```python
from build123d import *

# Parameters (mm, degrees)
SKETCH1_R                                            = 1.0000000000000033
SKETCH1_R_2                                          = 0.9999999999999979
SKETCH1_R_3                                          = 1.000000000000005
SKETCH1_R_4                                          = 1.0000000000000018
SKETCH1_R_5                                          = 1.0000000000000029
MAIN_BODY_DEPTH                                      = 10.5
PROFILE_STOPS_DEPTH                                  = 20
CSK_FOR_M3_HEX_SOCKET_COUNTERSUNK_HEAD_S_D           = 3.2
CSK_FOR_M3_HEX_SOCKET_COUNTERSUNK_HEAD_S_DEPTH       = 30.5
CSK_FOR_M3_HEX_SOCKET_COUNTERSUNK_HEAD_S_CSINK_D     = 6.94
CSK_FOR_M3_HEX_SOCKET_COUNTERSUNK_HEAD_S_CSINK_ANGLE = 90
CSK_FOR_M5_HEX_SOCKET_COUNTERSUNK_HEAD_S_D           = 5.3
CSK_FOR_M5_HEX_SOCKET_COUNTERSUNK_HEAD_S_DEPTH       = 30.5
CSK_FOR_M5_HEX_SOCKET_COUNTERSUNK_HEAD_S_CSINK_D     = 11.47
CSK_FOR_M5_HEX_SOCKET_COUNTERSUNK_HEAD_S_CSINK_ANGLE = 90
FILLET1_R                                            = 5
FILLET3_R                                            = 5
DRAFT1_ANGLE                                         = 0.5000000000000011
CHAMFER2_SIZE                                        = 0.5


with BuildPart() as part:
    # Sketch1 → Main Body (new body)
    with BuildSketch(Plane(origin=(0, 0, 0), x_dir=(1, 0, 0), z_dir=(0, 1, 0))):
        Polygon((-55, 0), (55, -6.74e-15), (-17.37778423417673, 103.36618828645003), align=None)
        with Locations(Location((-1.2076863300743388, 10.249999999999998, 0), (0, 0, 90))):
            Circle(SKETCH1_R, mode=Mode.SUBTRACT)
        with Locations(Location((23.307593201638067, 10.25, 0), (0, 0, 90))):
            Circle(SKETCH1_R_2, mode=Mode.SUBTRACT)
        with Locations(Location((-26.970095805737262, 47.04253374154206, 0), (0, 0, 90))):
            Circle(SKETCH1_R_3, mode=Mode.SUBTRACT)
        with Locations(Location((-18.585376386632234, 70.07936101399606, 0), (0, 0, 90))):
            Circle(SKETCH1_R_4, mode=Mode.SUBTRACT)
        with Locations(Location((2.578216537695586, 40.31670125636554, 0), (0, 0, 90))):
            Circle(SKETCH1_R_5, mode=Mode.SUBTRACT)
    extrude(amount=MAIN_BODY_DEPTH)

    # Sketch1<3> → Profile Stops (add)
    with BuildSketch(Plane(origin=(0, 0, 0), x_dir=(1, 0, 0), z_dir=(0, 1, 0))):
        Polygon((-55, 0), (-24.222965861786736, 0), (-24.22296586178674, 20.499999999999996), (40.64574546670092, 20.500000000000004), (-3.023529700877628, 82.86618828645001), (-25.209935646798243, 21.909538931178865), (-44.47363437290938, 28.920951869355026), align=None)
        Polygon((-7.671783462304414, 33.139573989716), (-10.559339294448062, 34.19055836239805), (-7.671783462304414, 42.1240528086273), (-7.6717834623044165, 50.56670125636553), (-4.598910728953966, 50.56670125636553), (-3.547926356271911, 53.45425708850919), (4.385568089957344, 50.56670125636554), (12.828216537695583, 50.56670125636554), (12.828216537695583, 47.49382852301509), (15.715772369839232, 46.44284415033304), (12.828216537695585, 38.5093497041038), (12.828216537695587, 30.066701256365544), (9.755343804345129, 30.066701256365544), (8.70435943166308, 27.1791454242219), (0.7708649854338496, 30.06670125636554), (-7.671783462304413, 30.06670125636554), align=None, mode=Mode.SUBTRACT)
    extrude(amount=-PROFILE_STOPS_DEPTH)

    # CSK for M3 Hex Socket Countersunk Head Screw1
    with Locations(Plane(origin=(-18.585376387, 10.5, -70.079361014), x_dir=(0, 0, 1), z_dir=(0, 1, 0))):
        with Locations((0, 0), (23.036827272, -8.384719419), (59.829361014, 41.892969589), (59.829361014, 17.377690057)):
            CounterSinkHole(CSK_FOR_M3_HEX_SOCKET_COUNTERSUNK_HEAD_S_D / 2, CSK_FOR_M3_HEX_SOCKET_COUNTERSUNK_HEAD_S_CSINK_D / 2, depth=CSK_FOR_M3_HEX_SOCKET_COUNTERSUNK_HEAD_S_DEPTH, counter_sink_angle=CSK_FOR_M3_HEX_SOCKET_COUNTERSUNK_HEAD_S_CSINK_ANGLE)

    # CSK for M5 Hex Socket Countersunk Head Screw1
    with Locations(Plane(origin=(2.578216538, 10.5, -40.316701256), x_dir=(0, 0, 1), z_dir=(0, 1, 0))):
        with Locations((0, 0)):
            CounterSinkHole(CSK_FOR_M5_HEX_SOCKET_COUNTERSUNK_HEAD_S_D / 2, CSK_FOR_M5_HEX_SOCKET_COUNTERSUNK_HEAD_S_CSINK_D / 2, depth=CSK_FOR_M5_HEX_SOCKET_COUNTERSUNK_HEAD_S_DEPTH, counter_sink_angle=CSK_FOR_M5_HEX_SOCKET_COUNTERSUNK_HEAD_S_CSINK_ANGLE)

    # Fillet1
    fillet1_edges = [part.edges().sort_by_distance(p)[0] for p in [
        (-55, -4.75, 0),
        (-24.222965861786736, -10, 0),
        (-44.47363437290938, -10, -28.920951869355026),
    ]]
    fillet(fillet1_edges, radius=FILLET1_R)

    # Fillet3
    fillet3_edges = [part.edges().sort_by_distance(p)[0] for p in [
        (55, 5.25, 6.74e-15),
        (-17.37778423417673, 5.25, -103.36618828645003),
        (-3.0235297008776296, -10, -82.86618828645001),
        (40.645745466700916, -10, -20.5),
    ]]
    fillet(fillet3_edges, radius=FILLET3_R)

    # Draft1
    draft1_faces = [part.faces().sort_by_distance(p)[0] for p in [
        (11.291780171020358, -10, -30.066701256365544),
        (9.229851618004107, -10, -28.62292334029372),
        (4.737612208548465, -10, -28.622923340293717),
        (-3.4504592384352817, -10, -30.06670125636554),
        (-7.671783462304413, -10.000000000000002, -31.60313762304077),
        (-9.115561378376238, -10, -33.665066176057024),
        (-9.115561378376238, -10, -38.157305585512674),
        (-6.135347095629191, -10, -50.56670125636553),
        (-7.671783462304415, -10, -46.345377032496415),
        (-4.073418542612939, -10, -52.010479172437364),
        (0.4188208668427172, -10, -52.010479172437364),
        (8.606892313826464, -10, -50.56670125636554),
        (12.828216537695583, -10, -49.030264889690315),
        (14.271994453767409, -10, -46.968336336674064),
        (14.271994453767409, -10, -42.476096927218414),
        (12.828216537695587, -10, -34.28802548023467),
    ]]
    draft(draft1_faces, Plane(origin=(0, 0, 0), x_dir=(0, 0, -1), z_dir=(0, -1, 0)), DRAFT1_ANGLE)

    # Chamfer2
    chamfer2_edges = [part.edges().sort_by_distance(p)[0] for p in [
        (-1.232085300572649, 10.5, 3.29e-15),
        (-36.61029010817967, 10.5, -50.52531267809811),
        (-51.95502018773441, 10.5, -2.1321178182447573),
        (18.811107882911628, 10.5, -51.683094143225006),
        (-16.61702500331109, 10.5, -97.58764822980864),
        (49.83014353103527, 10.5, -2.6912569338248247),
    ]]
    chamfer(chamfer2_edges, length=CHAMFER2_SIZE)


solid = part.part
```
The listing builds one solid part. Answer for the finished solid, in the listing's coordinates (mm). A direction names the side the tool comes from. Coordinates: 2 decimals unless noted, no trailing zeros. Write each loop counter-clockwise with the first axis right and the second up, starting at its lowest first coordinate (ties: lowest second). Pieces come first, ordered by that corner, then holes.
Q1. Section D-D, the plane y = 3 is taken. Write down the section's boundary in (x, z), then the cut area to 3 significant figures.
Returned:
outline: (-52.56, -6.71) - (-20.66, -94.34) arc R5 ccw to (-11.87, -95.5) - (49.49, -7.87) arc R5 ccw to (45.4, 0) - (-47.86, 0) arc R5 ccw to start; hole circle Ø3.2 at (-26.97, -47.04); hole circle Ø3.2 at (-18.59, -70.08); hole circle Ø3.2 at (-1.21, -10.25); hole circle Ø5.3 at (2.58, -40.32); hole circle Ø3.2 at (23.31, -10.25)
area: 5,580 mm2
Q2. Which of the six approach directions +Z, -Z, +X, -X, +Y, -Y give full straight-line access (tool end or side, diameter ignored) to faces 1 (the cylindrical face through (35.51, -10.14, -23.26)), 2 (the cylindrical face through (23.38, 4.25, -8.65)), 3 (the flat face through (10, 0, -11)), 4 (the cylindrical face through (-43.65, -10.14, -27.02)), 5 (the flat face through (-9, -20, -30))?
Returned:
face 1: +X, -Y
face 2: +Y, -Y
face 3: +Z, +X, -Y
face 4: -Z, -Y
face 5: +Z, -Z, +X, -X, -Y
Q3. Section C-C, the plane x = 33.5 is taken. Write down the section's boundary in (y, z), then the cut area to 3 significant figures.
Returned:
outline: (-20, -30.71) - (10, -30.71) - (10.5, -29.83) - (10.5, -0.5) - (10, 0) - (0, 0) - (0, -21.15) - (-20, -21.15) - close
area: 513 mm2
Q4. Section B-B, the plane z = -10.25 is taken. Write down the section's boundary in (x, y).
Returned:
outline: (-51.27, -20) - (-24.22, -20) - (-24.22, 0) - (-2.81, 0) - (-2.81, 8.63) - (-4.68, 10.5) - (-50.74, 10.5) - (-51.27, 10) - close; (0.39, 0) - (21.71, 0) - (21.71, 8.63) - (19.84, 10.5) - (2.26, 10.5) - (0.39, 8.63) - close; (24.91, 0) - (47.82, 0) - (47.82, 10) - (47.21, 10.5) - (26.78, 10.5) - (24.91, 8.63) - close
Q5. The mould has two halves that part along Z. Classify faces 6 (the conical face through (-25, 9, -47)), 7 (the cylindrical face through (-16.693, 5.07, -97.577)), 8 (the flat face through (-13, 10.5, -39)): released by +Z, released by -Z, zero draft, split by the parting line, or undercut.
Returned:
face 6: undercut
face 7: released by -Z
face 8: zero draft
Q6. Find the intervals of material crossed by line 1 along X through (y, z) = (2.75, -10.25); line 2 along Z through (x, y) = (4, -15); line 3 along X through (y, z) = (4, -10), in increasing order.
Returned:
line 1: x = -51.27 to -2.81, 0.39 to 21.71, 24.91 to 47.82
line 2: z = -72.84 to -50.85, -28.75 to -20.5
line 3: x = -51.36 to -2.79, 0.37 to 21.73, 24.89 to 48
Q7. Section A-A, the plane y = -12.5 is taken. Write down the section's boundary in (x, z).
Returned:
outline: (-52.56, -6.71) - (-46.18, -24.22) arc R5 ccw to (-39.78, -27.21) - (-25.21, -21.91) - (-6.31, -73.84) arc R5 ccw to (2.49, -75) - (35.14, -28.37) arc R5 ccw to (31.04, -20.5) - (-24.22, -20.5) - (-24.22, -5) arc R5 ccw to (-29.22, 0) - (-47.86, 0) arc R5 ccw to start; hole (-10.7, -34.13) - (-7.78, -42.14) - (-7.78, -50.68) - (-4.68, -50.68) - (-3.61, -53.59) - (4.4, -50.68) - (12.94, -50.68) - (12.94, -47.57) - (15.86, -46.51) - (12.94, -38.49) - (12.94, -29.96) - (9.83, -29.96) - (8.77, -27.04) - (0.75, -29.96) - (-7.78, -29.96) - (-7.78, -33.06) - close
Q8. Given P1, Ø4, axis at x = -18.59, z = -70.08, coming from the +Y side; P2, Ø12, axis at y = -9, z = -63.5, coming from the -X side; P3, Ø4, axis at x = -1.21, z = -10.25, coming from the -Y side; P4, Ø1.9, axis at x = -26.97, z = -47.04, coming from the +Y side, each flat-ended and moving along its own axis, determine where each tip first touches the part or whether it passes through.
Returned:
P1: stops at y = 9.03
P2: stops at x = -12.26
P3: stops at y = 0
P4: passes through
